Verification items for the finished model (mm, model axes). A direction names the side the tool comes from. Give positions to 0.01 mm unless a question says otherwise; leave off trailing zeros. Write each loop counter-clockwise with the first axis right and the second up, starting at its lowest first coordinate (ties: lowest second). Pieces come first, ordered by that corner, then holes. Notation, with made-up numbers: M 42.5,24 L 59.5,24 A36 ccw 59.5,62 Z; hole C 75.5,-29.75 d2. An arc over 180 degrees is marked long. Answer as a JSON object with one key per item and string values.
```python
from build123d import *

# Parameters (mm, degrees)
BOSS_EXTRU_1_DEPTH = 30


with BuildPart() as part:
    # Esquisse1 → Boss.-Extru.1 (new body)
    with BuildSketch(Plane.XY):
        Polygon((25, 20), (60, 40.207259422), (60, 0), (60, -15), (-60, -15), (-60, 0), (-60, 40.207259422), (-25, 20), (-25, 0), (25, 0), align=None)
        Polygon((30, 17.113248654), (55, 31.547005384), (55, 28.082903769), (30, 13.649147039), align=None, mode=Mode.SUBTRACT)
        Polygon((-30, 17.113248654), (-30, 13.649147039), (-55, 28.082903769), (-55, 31.547005384), align=None, mode=Mode.SUBTRACT)
    extrude(amount=BOSS_EXTRU_1_DEPTH)


solid = part.part
```
1) Section check B-B on z = 10.75. Record the boundary of the cut face in (x, y).
Completed:
{"outline": "M -60,-15 L 60,-15 L 60,40.21 L 25,20 L 25,0 L -25,0 L -25,20 L -60,40.21 Z; hole M -55,28.08 L -30,13.65 L -30,17.11 L -55,31.55 Z; hole M 30,13.65 L 55,28.08 L 55,31.55 L 30,17.11 Z"}
2) Access from +Z, -Z, +X, -X, +Y, -Y to the whole of each face (thin tool, end or side, straight path). Record for faces 1 (the face through (25, 10, 15)), 2 (the face through (1, -15, 15)), 3 (the face through (-42.675, 24.431, 14.79)).
Completed:
{"face 1": "+Z, -Z, +Y", "face 2": "+Z, -Z, +X, -X, -Y", "face 3": "+Z, -Z"}
3) Release check for a two-part mould opening along X. For faces 4 (the face through (1, -5, 0)), 5 (the face through (42.68, 20.97, 14.79)), 6 (the face through (-60, 13, 15)), 7 (the face through (60, 12, 15)) record: pulls with the +X half, pulls with the -X half, needs draft (parallel to the pull), parting line crosses it, or undercut.
Completed:
{"face 4": "needs draft", "face 5": "undercut", "face 6": "pulls with the -X half", "face 7": "pulls with the +X half"}
4) Section check D-D on y = 25.5. Record the boundary of the cut face in (x, z), and give its area (3 significant figures).
Completed:
{"outline": "M -60,0 L -50.53,0 L -50.53,30 L -60,30 Z; M -44.53,0 L -34.53,0 L -34.53,30 L -44.53,30 Z; M 34.53,0 L 44.53,0 L 44.53,30 L 34.53,30 Z; M 50.53,0 L 60,0 L 60,30 L 50.53,30 Z", "area": "1,170 mm2"}
5) Section check A-A on y = 6.5. Record the boundary of the cut face in (x, z).
Completed:
{"outline": "M -60,0 L -25,0 L -25,30 L -60,30 Z; M 25,0 L 60,0 L 60,30 L 25,30 Z"}
6) Section check C-C on x = 40.5. Record the boundary of the cut face in (y, z).
Completed:
{"outline": "M -15,0 L 19.71,0 L 19.71,30 L -15,30 Z; M 23.18,0 L 28.95,0 L 28.95,30 L 23.18,30 Z"}
7) Thickness scan on L1, parallel to X at y = 22.5, z = 7; L2, parallel to X at y = 20, z = 6; L3, parallel to X at y = 0.5, z = 12.5. Record the ranges inside material, lowest first.
Completed:
{"L1": "x = -60 to -45.33, -39.33 to -29.33, 29.33 to 39.33, 45.33 to 60", "L2": "x = -60 to -41, -35 to -25, 25 to 35, 41 to 60", "L3": "x = -60 to -25, 25 to 60"}
8) Go/stop test with flat-tipped pins: pin 1 (8 mm diameter, centred on x = 21.5, y = 24.5, fed in from +Z); pin 2 (10 mm diameter, centred on x = 11, z = 25.5, fed in from +Y); pin 3 (10 mm diameter, centred on x = -32.5, z = 8.5, fed in from +Y). Record where each tip stops, or that it passes through.
Completed:
{"pin 1": "passes through", "pin 2": "stops at y = 0", "pin 3": "stops at y = 27.22"}
